from build123d import *

# Parameters (mm, degrees)
ESQUISSE1_R             = 1.5
BOSS_EXTRU_1_DEPTH      = 7
ENL_V_MAT_EXTRU_1_REACH = 16.5
ESQUISSE2_W             = 12.350108933
ESQUISSE2_H             = 4
ESQUISSE3_R             = 3.25
BOSS_EXTRU_2_DEPTH      = 2


with BuildPart() as part:
    # Esquisse1 → Boss.-Extru.1 (new body)
    with BuildSketch(Plane(origin=(0, 0, 0), x_dir=(1, 0, 0), z_dir=(0, 1, 0))):
        Polygon((5.34048999, 9.25), (-5.34048999, 9.25), (-7.649891067, 5.25), (-20, 5.25), (-20, -5.25), (-7.649891067, -5.25), (-5.34048999, -9.25), (5.34048999, -9.25), (7.649891067, -5.25), (20, -5.25), (20, 5.25), (7.649891067, 5.25), align=None)
        with Locations((-15, 0)):
            Circle(ESQUISSE1_R, mode=Mode.SUBTRACT)
        with Locations((15, 0)):
            Circle(ESQUISSE1_R, mode=Mode.SUBTRACT)
        Polygon((6.062177826, 0), (3.031088913, 5.25), (-3.031088913, 5.25), (-6.062177826, 0), (-3.031088913, -5.25), (3.031088913, -5.25), align=None, mode=Mode.SUBTRACT)
    extrude(amount=BOSS_EXTRU_1_DEPTH)

    # Esquisse2 → Enlèv. mat.-Extru.1 (cut, up to next)
    with BuildSketch(Plane.XY.offset(5.25), mode=Mode.PRIVATE) as enl_v_mat_extru_1_sk1:
        with Locations((-13.824945533, 5)):
            Rectangle(ESQUISSE2_W, ESQUISSE2_H)
    enl_v_mat_extru_1_tool1 = extrude(enl_v_mat_extru_1_sk1.sketch, amount=-ENL_V_MAT_EXTRU_1_REACH, mode=Mode.PRIVATE) & part.part
    add(enl_v_mat_extru_1_tool1.solids().sort_by_distance((-13.824946, 5, 5.25))[0], mode=Mode.SUBTRACT)
    # Esquisse2 → Enlèv. mat.-Extru.1 (cut, up to next)
    with BuildSketch(Plane.XY.offset(5.25), mode=Mode.PRIVATE) as enl_v_mat_extru_1_sk2:
        with Locations((13.824945533, 5)):
            Rectangle(ESQUISSE2_W, ESQUISSE2_H)
    enl_v_mat_extru_1_tool2 = extrude(enl_v_mat_extru_1_sk2.sketch, amount=-ENL_V_MAT_EXTRU_1_REACH, mode=Mode.PRIVATE) & part.part
    add(enl_v_mat_extru_1_tool2.solids().sort_by_distance((13.824946, 5, 5.25))[0], mode=Mode.SUBTRACT)

    # Esquisse3 → Boss.-Extru.2 (add)
    with BuildSketch(Plane(origin=(0, 7, 0), x_dir=(1, 0, 0), z_dir=(0, 1, 0))):
        Polygon((-7.649891067, -5.25), (-7.649891067, 5.25), (-5.34048999, 9.25), (5.34048999, 9.25), (7.649891067, 5.25), (7.649891067, -5.25), (5.34048999, -9.25), (-5.34048999, -9.25), align=None)
        Circle(ESQUISSE3_R, mode=Mode.SUBTRACT)
    extrude(amount=BOSS_EXTRU_2_DEPTH)


solid = part.part
For this review, take the finished solid that the model builds, in its own axes (mm). A direction names the side the tool comes from. Round coordinates to 2 decimals unless told otherwise and drop trailing zeros. Loops run counter-clockwise (first coordinate to the right, second up) from the corner with the lowest first, then second, coordinate; pieces in that order, holes last. Notation, with made-up numbers: (-36.75, 63.5) - (-11.75, 63.5) arc R11 ccw to (-11.75, 78.5) - close; hole circle Ø11 at (64, -22). An arc over 180 degrees is marked (long way). One line per question, with ' | ' between items.
Q1. Take a section at A-A (x = 0). Give the boundary of the cut face in (y, z), and give its area (3 significant figures).
Taken from the geometry:
outline: (0, -9.25) - (9, -9.25) - (9, -3.25) - (7, -3.25) - (7, -5.25) - (0, -5.25) - close; (0, 5.25) - (7, 5.25) - (7, 3.25) - (9, 3.25) - (9, 9.25) - (0, 9.25) - close | area: 80.0 mm²
Q2. Take a section at B-B (y = 7.5). Give the boundary of the cut face in (x, z), and give its area (3 significant figures).
Taken from the geometry:
outline: (-7.65, -5.25) - (-5.34, -9.25) - (5.34, -9.25) - (7.65, -5.25) - (7.65, 5.25) - (5.34, 9.25) - (-5.34, 9.25) - (-7.65, 5.25) - close; hole circle Ø6.5 at (0, 0) | area: 231 mm²
Q3. The part is to be moulded in two halves that separate along Z. For faces 1 (the flat face through (6.48, 4.44, -7.28)), 2 (the flat face through (0, 4, 9.25)), 3 (the flat face through (4.525, 3.451, 2.662)), 4 (the flat face through (13.7, 3, 1.2)), say which applies: released by +Z, released by -Z, zero draft, split by the parting line, or undercut.
Taken from the geometry:
face 1: released by -Z | face 2: released by +Z | face 3: undercut | face 4: zero draft
Q4. Tool access review of faces 5 (the flat face through (7.65, 6, 0)), 6 (the flat face through (0, 3, 5.25)), 7 (the flat face through (14, 1, 5.25)), 8 (the flat face through (-7.65, 6, 0)), 9 (the flat face through (14, 1, -5.25)): name each direction out of +Z, -Z, +X, -X, +Y, -Y from which nothing blocks a thin tool from reaching the whole face with its end or side.
Taken from the geometry:
face 5: +Z, -Z, +X, +Y | face 6: -Y | face 7: +Z, +X, +Y, -Y | face 8: +Z, -Z, -X, +Y | face 9: -Z, +X, +Y, -Y
Q5. Take a section at C-C (z = 0.75). Give the boundary of the cut face in (x, y).
Taken from the geometry:
outline: (-20, 0) - (-16.3, 0) - (-16.3, 3) - (-20, 3) - close; (-13.7, 0) - (-5.63, 0) - (-5.63, 7) - (-3.16, 7) - (-3.16, 9) - (-7.65, 9) - (-7.65, 3) - (-13.7, 3) - close; (3.16, 7) - (5.63, 7) - (5.63, 0) - (13.7, 0) - (13.7, 3) - (7.65, 3) - (7.65, 9) - (3.16, 9) - close; (16.3, 0) - (20, 0) - (20, 3) - (16.3, 3) - close
Q6. For pin 1 (2.5 mm diameter, centred on x = -13, y = 2, fed in from +Z); pin 2 (4 mm diameter, centred on y = 7, z = -2.5, fed in from +X); pin 3 (5 mm diameter, centred on x = -15.5, z = -2.5, fed in from +Y), all flat-tipped, find the tip position at first contact; note any pin that passes through.
Taken from the geometry:
pin 1: stops at z = 5.25 | pin 2: stops at x = 7.65 | pin 3: stops at y = 3
Q7. For line 1 along X through (y, z) = (2, 0); line 2 along Z through (x, y) = (3, 2.75); line 3 along Z through (x, y) = (-15, 1.4), list the stretches that pass through material, from the lowest coordinate up. Write a range as [from, to].
Taken from the geometry:
line 1: x = [-20, -16.5], [-13.5, -6.06], [6.06, 13.5], [16.5, 20] | line 2: z = [-9.25, -5.25], [5.25, 9.25] | line 3: z = [-5.25, -1.5], [1.5, 5.25]
Q8. Take a section at D-D (y = 1.25). Give the boundary of the cut face in (x, z), and give its area (3 significant figures).
Taken from the geometry:
outline: (-20, -5.25) - (-7.65, -5.25) - (-5.34, -9.25) - (5.34, -9.25) - (7.65, -5.25) - (20, -5.25) - (20, 5.25) - (7.65, 5.25) - (5.34, 9.25) - (-5.34, 9.25) - (-7.65, 5.25) - (-20, 5.25) - close; hole circle Ø3 at (-15, 0); hole (-6.06, 0) - (-3.03, -5.25) - (3.03, -5.25) - (6.06, 0) - (3.03, 5.25) - (-3.03, 5.25) - close; hole circle Ø3 at (15, 0) | area: 414 mm²
